```python
from build123d import *

# Parameters (mm, degrees)
SKETCH1_R           = 22.5
SKETCH1_R_2         = 2.5
BOSS_EXTRUDE1_DEPTH = 4
SKETCH2_R           = 7.05
SKETCH2_R_2         = 4.05
BOSS_EXTRUDE2_DEPTH = 18
SKETCH3_R           = 1.65
CUT_EXTRUDE1_DEPTH  = 9
SKETCH4_R           = 10
SKETCH4_R_2         = 7
BOSS_EXTRUDE3_DEPTH = 5


with BuildPart() as part:
    # Sketch1 → Boss-Extrude1 (new body)
    with BuildSketch(Plane(origin=(0, 0, 0), x_dir=(1, 0, 0), z_dir=(0, 1, 0))):
        with Locations(Location((0, 0, 0), (0, 0, 270))):
            Circle(SKETCH1_R)
        with Locations(Location((-12.374368671, 12.374368671, 0), (0, 0, 270))):
            Circle(SKETCH1_R_2, mode=Mode.SUBTRACT)
        with Locations(Location((12.374368671, 12.374368671, 0), (0, 0, 270))):
            Circle(SKETCH1_R_2, mode=Mode.SUBTRACT)
        with Locations(Location((12.374368671, -12.374368671, 0), (0, 0, 270))):
            Circle(SKETCH1_R_2, mode=Mode.SUBTRACT)
        with Locations(Location((-12.374368671, -12.374368671, 0), (0, 0, 270))):
            Circle(SKETCH1_R_2, mode=Mode.SUBTRACT)
    extrude(amount=BOSS_EXTRUDE1_DEPTH)

    # Sketch2 → Boss-Extrude2 (add)
    with BuildSketch(Plane(origin=(0, 4, 0), x_dir=(1, 0, 0), z_dir=(0, 1, 0))):
        with Locations(Location((0, 0, 0), (0, 0, 270))):
            Circle(SKETCH2_R)
        with Locations(Location((0, 0, 0), (0, 0, 270))):
            Circle(SKETCH2_R_2, mode=Mode.SUBTRACT)
    extrude(amount=BOSS_EXTRUDE2_DEPTH)

    # Sketch3 → Cut-Extrude1 (cut, symmetric)
    with BuildSketch(Plane.XY):
        with Locations((0, 14.5)):
            Circle(SKETCH3_R)
    extrude(amount=CUT_EXTRUDE1_DEPTH, both=True, mode=Mode.SUBTRACT)

    # Sketch4 → Boss-Extrude3 (add)
    with BuildSketch(Plane(origin=(0, 4, 0), x_dir=(1, 0, 0), z_dir=(0, 1, 0))):
        with Locations(Location((0, 0, 0), (0, 0, 270))):
            Circle(SKETCH4_R)
        Circle(SKETCH4_R_2, mode=Mode.SUBTRACT)
    extrude(amount=BOSS_EXTRUDE3_DEPTH)


solid = part.part
```
Check sheet for the modelled part. Datum: model origin and axes. Units: mm. A direction names the side the tool comes from. Give positions to 0.01 mm unless a question says otherwise; leave off trailing zeros. Order: outer loops, then holes, each group sorted by start corner. A loop starts at its lowest first (then second) coordinate and runs counter-clockwise, first axis right, second up. Notation, with made-up numbers: (2.5, 36) -> (58.5, 36) arc R17 cw to (58.5, 61) -> close; hole circle Ø8 at (-27.75, -14). An arc over 180 degrees is marked (long way). Use CSV: the item, a comma, the result in double quotes. Start each with the question number.
1) Sectioned sample at C-C, the plane y = 14.5. Record the boundary of the cut face in (x, z).
2) Mould release check, pull along Z, two halves, no side actions. Record for faces 3 (the face through (-8.618, 1.972, 20.784)), 4 (the face through (-1.65, 14.57, 5.4)), 5 (the face through (9.934, 1.972, 11.832)): released by +Z, released by -Z, zero draft, split by the parting line, or undercut.
3) Sectioned sample at A-A, the plane x = 0. Record the boundary of the cut face in (y, z).
4) Material ranges on line 1 (X direction, y = 15.75, z = 0); line 2 (X direction, y = 3.75, z = -12), recorded low to high. Write a range as from..to.
5) Sectioned sample at B-B, the plane z = 0. Record the boundary of the cut face in (x, y), plus the area to 4 significant figures.
6) Set-up check for faces 1 (the face through (-9.76, 6.46, -2.17)), 2 (the face through (-11.62, 1.97, -9.99)): record each of +Z, -Z, +X, -X, +Y, -Y from which the full face is reachable in a straight line by a thin tool's end or side.
7) Sectioned sample at D-D, the plane y = 19.5. Record the boundary of the cut face in (x, z).
8) Go/stop test with flat-tipped pins: P1, Ø6.5, axis at x = 0, z = 0, coming from the +Y side; P2, Ø3, axis at x = 9, y = 13, coming from the -Z side; P3, Ø8, axis at y = 18.5, z = -9.5, coming from the +X side; P4, Ø4, axis at x = 0, y = 14.5, coming from the -Z side. Record where each tip stops, or that it passes through.
Recorded:
1,outline,"(-1.65, -6.85) -> (-1.65, -3.7) arc R4.05 cw to (-1.65, 3.7) -> (-1.65, 6.85) arc R7.05 ccw to start; (1.65, -6.85) arc R7.05 ccw to (1.65, 6.85) -> (1.65, 3.7) arc R4.05 cw to (1.65, -3.7) -> close"
2,face 3,"split by the parting line"
2,face 4,"zero draft"
2,face 5,"undercut"
3,outline,"(0, -22.5) -> (4, -22.5) -> (4, -10) -> (9, -10) -> (9, -7.05) -> (12.85, -7.05) -> (12.85, -4.05) -> (4, -4.05) -> (4, 4.05) -> (12.85, 4.05) -> (12.85, 7.05) -> (9, 7.05) -> (9, 10) -> (4, 10) -> (4, 22.5) -> (0, 22.5) -> close; (16.15, -7.05) -> (22, -7.05) -> (22, -4.05) -> (16.15, -4.05) -> close; (16.15, 4.05) -> (22, 4.05) -> (22, 7.05) -> (16.15, 7.05) -> close"
4,line 1,"-7.05..-4.05, 4.05..7.05"
4,line 2,"-19.03..-14.85, -9.9..9.9, 14.85..19.03"
5,outline,"(-22.5, 0) -> (22.5, 0) -> (22.5, 4) -> (10, 4) -> (10, 9) -> (7.05, 9) -> (7.05, 22) -> (4.05, 22) -> (4.05, 4) -> (-4.05, 4) -> (-4.05, 22) -> (-7.05, 22) -> (-7.05, 9) -> (-10, 9) -> (-10, 4) -> (-22.5, 4) -> close"
5,area,"317.5 mm2"
6,face 1,"+Y"
6,face 2,"+Y, -Y"
7,outline,"circle Ø14.1 at (0, 0); hole circle Ø8.1 at (0, 0)"
8,P1,"y = 4"
8,P2,"through"
8,P3,"x = 4.41"
8,P4,"z = -7.05"
